Can you work these out from the model? Positions are in its coordinate system, mm. Face numbers are marked on the shaded views. A direction names the side the tool comes from. Round coordinates to 2 decimals unless told otherwise and drop trailing zeros. Loops run counter-clockwise (first coordinate to the right, second up) from the corner with the lowest first, then second, coordinate; pieces in that order, holes last. Notation, with made-up numbers: (-12.75, 37) -> (16.25, 37) arc R13 cw to (16.25, 41) -> close; hole circle Ø8 at (39.25, -37). An arc over 180 degrees is marked (long way). Answer as a JSON object with one key per item and string values.
```python
from build123d import *
from build123d.topology import SkipClean

# Parameters (mm, degrees)
BOSS_EXTRUDE1_DEPTH     = 52
SHELL1_START            = 3
SHELL1_DEPTH            = 46
SKETCH2_R               = 4.5
BOSS_EXTRUDE2_DEPTH     = 52
SKETCH3_R               = 3.25
CUT_EXTRUDE1_DEPTH      = 49
SKETCH4_R               = 1.7
CUT_EXTRUDE2_DEPTH      = 91.166512631
CUT_EXTRUDE3_DEPTH      = 20
CUT_EXTRUDE3_DEPTH_BACK = 20
CUT_EXTRUDE4_DEPTH      = 3.5
SKETCH7_R               = 4
CUT_EXTRUDE5_DEPTH      = 3.5
SKETCH8_W               = 6
SKETCH8_H               = 20
BOSS_EXTRUDE3_DEPTH     = 8
SKETCH9_W               = 1.9
SKETCH9_H               = 16.6
CUT_EXTRUDE6_DEPTH      = 6
SKETCH10_R              = 15
SKETCH10_R_2            = 9.1
BOSS_EXTRUDE4_DEPTH     = 8
SKETCH11_R              = 9.1
CUT_EXTRUDE7_DEPTH      = 3.5


# Read off the part's stored shape, not the designer's step: Shell1
with BuildPart() as part:
    # Sketch1 → Boss-Extrude1 (new body)
    with BuildSketch(Plane.XY):
        with BuildLine():
            Line((-45, -55), (45, -55))
            ThreePointArc((45, -55), (52.071067812, -52.071067812), (55, -45))
            Line((55, -45), (55, -10))
            ThreePointArc((55, -10), (52.071067812, -2.928932188), (45, 0))
            Line((45, 0), (-45, 0))
            ThreePointArc((-45, 0), (-52.071067812, -2.928932188), (-55, -10))
            Line((-55, -10), (-55, -45))
            ThreePointArc((-55, -45), (-52.071067812, -52.071067812), (-45, -55))
        make_face()
    extrude(amount=BOSS_EXTRUDE1_DEPTH)

    # Shell1 outline → Shell1 (cut)
    with BuildSketch(Plane.XY.offset(SHELL1_START)):
        with BuildLine():
            Line((45, -3), (45, 0))
            Line((45, 0), (-45, 0))
            Line((-45, 0), (-45, -3))
            ThreePointArc((-45, -3), (-49.949747468, -5.050252532), (-52, -10))
            Line((-52, -10), (-52, -45))
            ThreePointArc((-52, -45), (-49.949747468, -49.949747468), (-45, -52))
            Line((-45, -52), (45, -52))
            ThreePointArc((45, -52), (49.949747468, -49.949747468), (52, -45))
            Line((52, -45), (52, -10))
            ThreePointArc((52, -10), (49.949747468, -5.050252532), (45, -3))
        make_face()
    extrude(amount=SHELL1_DEPTH, mode=Mode.SUBTRACT)

    # Sketch2 → Boss-Extrude2 (add)
    with BuildSketch(Plane(origin=(0, 0, 0), x_dir=(1, 0, 0), z_dir=(0, 1, 0))):
        with Locations(Location((-40, -8, 0), (0, 0, 270))):
            Circle(SKETCH2_R)
        with Locations(Location((40, -8, 0), (0, 0, 270))):
            Circle(SKETCH2_R)
        with Locations(Location((-40, -40, 0), (0, 0, 270))):
            Circle(SKETCH2_R)
        with Locations(Location((40, -40, 0), (0, 0, 270))):
            Circle(SKETCH2_R)
    extrude(amount=-BOSS_EXTRUDE2_DEPTH)

    # Sketch3 → Cut-Extrude1 (cut)
    with BuildSketch(Plane.XZ.offset(55)):
        with Locations(Location((-40, 8, 0), (0, 0, 270))):
            Circle(SKETCH3_R)
        with Locations(Location((40, 8, 0), (0, 0, 270))):
            Circle(SKETCH3_R)
        with Locations(Location((-40, 40, 0), (0, 0, 270))):
            Circle(SKETCH3_R)
        with Locations(Location((40, 40, 0), (0, 0, 270))):
            Circle(SKETCH3_R)
    extrude(amount=-CUT_EXTRUDE1_DEPTH, mode=Mode.SUBTRACT)

    # Sketch4 → Cut-Extrude2 (cut, through all)
    with BuildSketch(Plane.XZ.offset(6)):
        with Locations(Location((-40, 8, 0), (0, 0, 270))):
            Circle(SKETCH4_R)
        with Locations(Location((40, 8, 0), (0, 0, 270))):
            Circle(SKETCH4_R)
        with Locations(Location((-40, 40, 0), (0, 0, 270))):
            Circle(SKETCH4_R)
        with Locations(Location((40, 40, 0), (0, 0, 270))):
            Circle(SKETCH4_R)
    extrude(amount=-CUT_EXTRUDE2_DEPTH, mode=Mode.SUBTRACT)

    # Sketch5 → Cut-Extrude3 (cut, two sides: drawn at the far end of the back side and taken through both)
    with BuildSketch(Plane.XY.offset(26).offset(-CUT_EXTRUDE3_DEPTH_BACK)):
        Polygon((-51, -14), (-51, -11.5), (-55.5, -16), (-55.5, -18.5), align=None)
        Polygon((51, -14), (51, -11.5), (55.5, -16), (55.5, -18.5), align=None)
        Polygon((-51, -20), (-51, -17.5), (-55.5, -22), (-55.5, -24.5), align=None)
        Polygon((51, -20), (51, -17.5), (55.5, -22), (55.5, -24.5), align=None)
        Polygon((-51, -26), (-51, -23.5), (-55.5, -28), (-55.5, -30.5), align=None)
        Polygon((51, -26), (51, -23.5), (55.5, -28), (55.5, -30.5), align=None)
        Polygon((-51, -32), (-51, -29.5), (-55.5, -34), (-55.5, -36.5), align=None)
        Polygon((51, -32), (51, -29.5), (55.5, -34), (55.5, -36.5), align=None)
        Polygon((-51, -38), (-51, -35.5), (-55.5, -40), (-55.5, -42.5), align=None)
        Polygon((51, -38), (51, -35.5), (55.5, -40), (55.5, -42.5), align=None)
    extrude(amount=CUT_EXTRUDE3_DEPTH + CUT_EXTRUDE3_DEPTH_BACK, mode=Mode.SUBTRACT)

    # Sketch6 → Cut-Extrude4 (cut)
    with BuildSketch(Plane.XZ.offset(55)):
        with BuildLine():
            Line((-34.5, 12), (-34.5, 40))
            ThreePointArc((-34.5, 40), (-33, 41.5), (-31.5, 40))
            Line((-31.5, 40), (-31.5, 12))
            ThreePointArc((-31.5, 12), (-33, 10.5), (-34.5, 12))
        make_face()
        with BuildLine():
            Line((-28.5, 12), (-28.5, 40))
            ThreePointArc((-28.5, 40), (-27, 41.5), (-25.5, 40))
            Line((-25.5, 40), (-25.5, 12))
            ThreePointArc((-25.5, 12), (-27, 10.5), (-28.5, 12))
        make_face()
        with BuildLine():
            Line((-22.5, 12), (-22.5, 40))
            ThreePointArc((-22.5, 40), (-21, 41.5), (-19.5, 40))
            Line((-19.5, 40), (-19.5, 12))
            ThreePointArc((-19.5, 12), (-21, 10.5), (-22.5, 12))
        make_face()
        with BuildLine():
            Line((-16.5, 12), (-16.5, 40))
            ThreePointArc((-16.5, 40), (-15, 41.5), (-13.5, 40))
            Line((-13.5, 40), (-13.5, 12))
            ThreePointArc((-13.5, 12), (-15, 10.5), (-16.5, 12))
        make_face()
        with BuildLine():
            Line((-10.5, 12), (-10.5, 40))
            ThreePointArc((-10.5, 40), (-9, 41.5), (-7.5, 40))
            Line((-7.5, 40), (-7.5, 12))
            ThreePointArc((-7.5, 12), (-9, 10.5), (-10.5, 12))
        make_face()
        with BuildLine():
            Line((-4.5, 12), (-4.5, 40))
            ThreePointArc((-4.5, 40), (-3, 41.5), (-1.5, 40))
            Line((-1.5, 40), (-1.5, 12))
            ThreePointArc((-1.5, 12), (-3, 10.5), (-4.5, 12))
        make_face()
        with BuildLine():
            Line((31.5, 12), (31.5, 40))
            ThreePointArc((31.5, 40), (33, 41.5), (34.5, 40))
            Line((34.5, 40), (34.5, 12))
            ThreePointArc((34.5, 12), (33, 10.5), (31.5, 12))
        make_face()
    extrude(amount=-CUT_EXTRUDE4_DEPTH, mode=Mode.SUBTRACT)

    # Sketch7 → Cut-Extrude5 (cut)
    with BuildSketch(Plane(origin=(0, 0, 0), x_dir=(-1, 0, 0), z_dir=(0, 0, -1))):
        with Locations((30, -12)):
            Circle(SKETCH7_R)
        with Locations((-30, -12)):
            Circle(SKETCH7_R)
    extrude(amount=-CUT_EXTRUDE5_DEPTH, mode=Mode.SUBTRACT)

    # Sketch8 → Boss-Extrude3 (add)
    with BuildSketch(Plane(origin=(0, -52, 0), x_dir=(1, 0, 0), z_dir=(0, 1, 0))):
        with Locations((-44, -26)):
            Rectangle(SKETCH8_W, SKETCH8_H)
    extrude(amount=BOSS_EXTRUDE3_DEPTH)

    # Sketch9 → Cut-Extrude6 (cut)
    with BuildSketch(Plane(origin=(0, -44, 0), x_dir=(1, 0, 0), z_dir=(0, 1, 0))):
        with Locations((-44, -26)):
            Rectangle(SKETCH9_W, SKETCH9_H)
    extrude(amount=-CUT_EXTRUDE6_DEPTH, mode=Mode.SUBTRACT)

    # Sketch10 → Boss-Extrude4 (add)
    with BuildSketch(Plane(origin=(0, -52, 0), x_dir=(1, 0, 0), z_dir=(0, 1, 0))):
        with Locations(Location((15, -26, 0), (0, 0, 270))):
            Circle(SKETCH10_R)
        with Locations(Location((15, -26, 0), (0, 0, 270))):
            Circle(SKETCH10_R_2, mode=Mode.SUBTRACT)
    extrude(amount=BOSS_EXTRUDE4_DEPTH)

    # Sketch11 → Cut-Extrude7 (cut)
    with SkipClean():  # the faces are left unmerged after this step: merging them gives an invalid solid
        with BuildSketch(Plane.XZ.offset(55)):
            with Locations(Location((15, 26, 0), (0, 0, 270))):
                Circle(SKETCH11_R)
        extrude(amount=-CUT_EXTRUDE7_DEPTH, mode=Mode.SUBTRACT)


solid = part.part
```
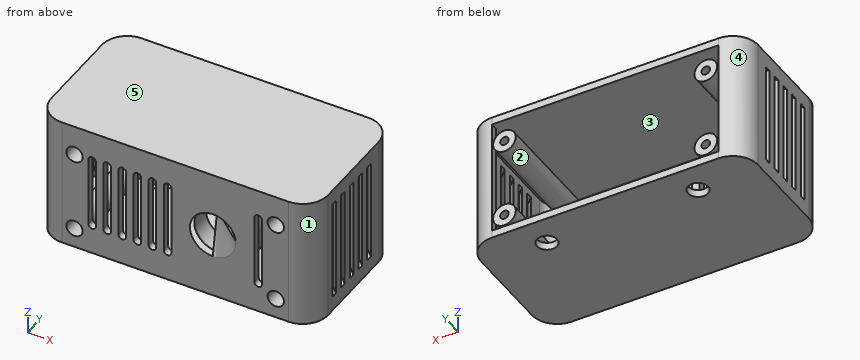
Q1. I'm going to push flat-ended pins straight in: pin 1 (3.5 mm diameter, centred on y = -53, z = 32.5, fed in from -X); pin 2 (8 mm diameter, centred on y = -8, z = 40.5, fed in from -X); pin 3 (2.5 mm diameter, centred on x = -40, z = 40, fed in from -Y); pin 4 (1.8 mm diameter, centred on y = -47.5, z = 22, fed in from +X). Where does each tip first touch, or does it pass through?
Determined:
{"pin 1": "x = -52.81", "pin 2": "x = -55", "pin 3": "through", "pin 4": "x = 54.87"}
Q2. I want a section at A-A, the plane x = -15. Write out the boundary of the cut face in (y, z).
Determined:
{"outline": "(-55, 0) -> (0, 0) -> (0, 3) -> (-52, 3) -> (-52, 10.5) -> (-55, 10.5) -> close; (-55, 41.5) -> (-52, 41.5) -> (-52, 49) -> (0, 49) -> (0, 52) -> (-55, 52) -> close"}
Q3. If I drill on L1, parallel to X at y = -45.5, z = 26; L2, parallel to Z at x = 7.5, y = -11.5; L3, parallel to X at y = -4.2, z = 8, over which ranges is the centre line in solid material (lowest first)? Write a range as [from, to].
Determined:
{"L1": "[-54.99, -51.98], [-47, -44.95], [-43.05, -41], [0, 5.9], [24.1, 30], [51.98, 54.99]", "L2": "[0, 3], [49, 52]", "L3": "[-53.15, -48.92], [-44.5, -41.7], [-38.3, -35.5], [35.5, 38.3], [41.7, 44.5], [48.92, 53.15]"}
Q4. We'd pull the mould along Z, two halves only. Please class the marked faces 3, 4 and 5: pulls with the +Z half, pulls with the -Z half, needs draft (parallel to the pull), parting line crosses it, or undercut.
Determined:
{"face 3": "undercut", "face 4": "needs draft", "face 5": "pulls with the +Z half"}
Q5. I want a section at B-B, the plane y = -4.5. Give the number of separate pieces and of enclosed holes in the cut face, then the cut area to 3 significant figures.
Determined:
{"separate pieces": "5", "enclosed holes": "5", "area": "1,230 mm²"}
Q6. On a 3-axis mill with a long thin cutter (end or side, diameter ignored), from which of +Z, -Z, +X, -X, +Y, -Y can I reach the whole of each face in a straight line? I mean the marked faces 1 and 2. Say none if no direction works.
Determined:
{"face 1": "+Z, -Z, +X, -Y", "face 2": "+Y"}
